Model file for the job. Use its own axes, mm. A direction names the side the tool comes from. Coordinates: 2 decimals unless noted, no trailing zeros. Order: outer loops, then holes, each group sorted by start corner. A loop starts at its lowest first (then second) coordinate and runs counter-clockwise, first axis right, second up.
from build123d import *

# Parameters (mm, degrees)
SKETCH_1_R          = 60
EXTRUDE_1_DEPTH     = 10
CHAMFER_1_SIZE      = 0.961662122
CHAMFER_1_SIZE_2    = 1
SKETCH_2_R          = 6
CUT_EXTRUDE_1_DEPTH = 10


with BuildPart() as part:
    # 草图1 → 凸台-拉伸1 (new body)
    with BuildSketch(Plane.XY):
        Circle(SKETCH_1_R)
        with BuildLine():
            Line((-38.547540209, 35.446506114), (-37.123106012, 34.236311133))
            ThreePointArc((-37.123106012, 34.236311133), (-50.5, 0), (-37.123106012, -34.236311133))
            Line((-37.123106012, -34.236311133), (-38.547540209, -35.446506114))
            ThreePointArc((-38.547540209, -35.446506114), (-38.678740931, -38.678740931), (-35.446506114, -38.547540209))
            Line((-35.446506114, -38.547540209), (-34.236311133, -37.123106012))
            ThreePointArc((-34.236311133, -37.123106012), (0, -50.5), (34.236311133, -37.123106012))
            Line((34.236311133, -37.123106012), (35.446506114, -38.547540209))
            ThreePointArc((35.446506114, -38.547540209), (38.678740931, -38.678740931), (38.547540209, -35.446506114))
            Line((38.547540209, -35.446506114), (37.123106012, -34.236311133))
            ThreePointArc((37.123106012, -34.236311133), (50.5, 0), (37.123106012, 34.236311133))
            Line((37.123106012, 34.236311133), (38.547540209, 35.446506114))
            ThreePointArc((38.547540209, 35.446506114), (38.678740931, 38.678740931), (35.446506114, 38.547540209))
            Line((35.446506114, 38.547540209), (34.236311133, 37.123106012))
            ThreePointArc((34.236311133, 37.123106012), (0, 50.5), (-34.236311133, 37.123106012))
            Line((-34.236311133, 37.123106012), (-35.446506114, 38.547540209))
            ThreePointArc((-35.446506114, 38.547540209), (-38.678740931, 38.678740931), (-38.547540209, 35.446506114))
        make_face(mode=Mode.SUBTRACT)
    extrude(amount=EXTRUDE_1_DEPTH)

    # 倒角1
    # the kernel refuses this chamfer: 1, 0.961662122 mm, written as the material it takes off along each edge
    with BuildSketch(Plane(origin=(34.236311133, 37.123106012, -2.597741643), x_dir=(-0.7418547410377812, 0.6705606185869901, 0), z_dir=(0, 0, 1)), Plane(origin=(-37.123106012, 34.236311133, -2.597741643), x_dir=(-0.6705606185869967, -0.741854741037775, 0), z_dir=(0, 0, 1)), Plane(origin=(-34.236311133, -37.123106012, -2.597741643), x_dir=(0.7418547410378011, -0.670560618586968, 0), z_dir=(0, 0, 1)), Plane(origin=(37.123106012, -34.236311133, -2.597741643), x_dir=(0.6705606185869861, 0.7418547410377846, 0), z_dir=(0, 0, 1))) as chamfer_1_piece_1:
        with BuildLine():
            Line((1.010153596, 0), (CHAMFER_1_SIZE * 0.0306993646522, -CHAMFER_1_SIZE * 0.999528663409))
            Line((CHAMFER_1_SIZE * 0.0306993646522, -CHAMFER_1_SIZE * 0.999528663409), (0, 0))
            ThreePointArc((0, 0), (0.519364344, -0.00252381), (1.010153596, 0))
        make_face()
    extrude(amount=15.195483286, mode=Mode.SUBTRACT)
    with BuildSketch(Plane(origin=(-34.236311133, 37.123106012, -2.571682988), x_dir=(-0.6474700896278034, 0.7620908627174087, 0), z_dir=(0, 0, 1)), Plane(origin=(-37.123106012, -34.236311133, -2.571682988), x_dir=(-0.7620908627174083, -0.6474700896278041, 0), z_dir=(0, 0, 1)), Plane(origin=(34.236311133, -37.123106012, -2.571682988), x_dir=(0.6474700896277805, -0.7620908627174282, 0), z_dir=(0, 0, 1)), Plane(origin=(37.123106012, 34.236311133, -2.571682988), x_dir=(0.7620908627174152, 0.6474700896277957, 0), z_dir=(0, 0, 1))) as chamfer_1_piece_2:
        with BuildLine():
            Line((CHAMFER_1_SIZE_2, 0), (0.030170276, -0.969829724))
            ThreePointArc((0.030170276, -0.969829724), (0.017838593, -0.498535983), (0, 0))
            Line((0, 0), (CHAMFER_1_SIZE_2, 0))
        make_face()
    extrude(amount=15.143365976, mode=Mode.SUBTRACT)

    # 草图2 → 切除-拉伸1 (cut)
    with BuildSketch(Plane(origin=(0, 0, 0), x_dir=(-1, 0, 0), z_dir=(0, 0, -1))):
        with Locations((60, 0)):
            Circle(SKETCH_2_R)
        with Locations((-60, 0)):
            Circle(SKETCH_2_R)
        with Locations((0, -60)):
            Circle(SKETCH_2_R)
        with Locations((0, 60)):
            Circle(SKETCH_2_R)
    extrude(amount=-CUT_EXTRUDE_1_DEPTH, mode=Mode.SUBTRACT)

    # 倒角2
    # the kernel refuses this chamfer: 2, 1.907033604 mm, written as the material it takes off along each edge
    with BuildSketch(Plane(origin=(-5.992495307, 59.7, 16.798280923), x_dir=(-0.9933125969799259, -0.11545598590369961, 0), z_dir=(0, 0, -1)), Plane(origin=(59.7, 5.992495307, 16.798280923), x_dir=(-0.11545598590369978, 0.9933125969799259, 0), z_dir=(0, 0, -1)), Plane(origin=(5.992495307, -59.7, 16.798280923), x_dir=(0.993312596979926, 0.11545598590369918, 0), z_dir=(0, 0, -1)), Plane(origin=(-59.7, -5.992495307, 16.798280923), x_dir=(0.11545598590370064, -0.9933125969799258, 0), z_dir=(0, 0, -1))) as chamfer_2_piece_1:
        with BuildLine():
            Line((1.880602566, 0), (-0.414776487, -2.618663345))
            ThreePointArc((-0.414776487, -2.618663345), (-0.066481971, -1.366902402), (0, 0))
            ThreePointArc((0, 0), (0.966657818, 0.007362718), (1.880602566, 0))
        make_face()
    extrude(amount=23.596561846, mode=Mode.SUBTRACT)
    with BuildSketch(Plane(origin=(5.992495307, 59.7, 16.798280923), x_dir=(0.9933125969799259, -0.11545598590369989, 0), z_dir=(0, 0, -1))) as chamfer_2_piece_2:
        with BuildLine():
            Line((1.880602566, 0), (-0.414776487, 2.618663345))
            ThreePointArc((-0.414776487, 2.618663345), (-0.066481971, 1.366902402), (0, 0))
            ThreePointArc((0, 0), (0.966657818, -0.007362718), (1.880602566, 0))
        make_face()
    extrude(amount=23.596561846, mode=Mode.SUBTRACT)
    with BuildSketch(Plane(origin=(-5.992495307, -59.7, 16.798280923), x_dir=(0.26943037499341854, 0.9630198715659537, 0), z_dir=(0, 0, -1)), Plane(origin=(59.7, -5.992495307, 16.798280923), x_dir=(-0.963019871565954, 0.26943037499341704, 0), z_dir=(0, 0, -1)), Plane(origin=(-59.7, 5.992495307, 16.798280923), x_dir=(0.9630198715659543, -0.26943037499341643, 0), z_dir=(0, 0, -1))) as chamfer_2_piece_3:
        with BuildLine():
            Line((2.651308592, 0), (-0.294205559, -1.857446931))
            ThreePointArc((-0.294205559, -1.857446931), (-0.158498115, -0.953603635), (0, 0))
            ThreePointArc((0, 0), (1.360472479, -0.148177801), (2.651308592, 0))
        make_face()
    extrude(amount=23.596561846, mode=Mode.SUBTRACT)


solid = part.part
Q1. Cut at A-A, the plane x = 0. List the corners of the cut face in (y, z), plus the area to 3 significant figures.
Established:
outline: (-54, 0) - (-50.5, 0) - (-50.5, 10) - (-54, 10) - close; (50.5, 0) - (54, 0) - (54, 10) - (50.5, 10) - close
area: 70.0 mm2
Q2. Which spindle directions (+Z, -Z, +X, -X, +Y, -Y) get a long thin tool onto all of the face, cutting with end or side? Do faces 1 (the face through (58.3, -6.55, 5.07)), 2 (the face through (6.587, 58.331, 5.07)), 3 (the face through (42.04, -42.81, 4.93)), 4 (the face through (0.493, 50.498, 4.93)), 5 (the face through (6.587, -58.331, 5.07)). Say none if no direction does.
Established:
face 1: +Z, -Z, +X
face 2: +Z, -Z, +Y
face 3: +Z, -Z, +X, -Y
face 4: +Z, -Z
face 5: +Z, -Z, -Y
Q3. Cut at B-B, the plane y = -28.5. List the corners of the cut face in (x, z), plus the area to 3 significant figures.
Established:
outline: (-52.8, 0) - (-41.69, 0) - (-41.69, 10) - (-52.8, 10) - close; (41.69, 0) - (52.8, 0) - (52.8, 10) - (41.69, 10) - close
area: 222 mm2
Q4. Mould opens along Y. For faces 6 (the face through (-54, 0, 5)), 7 (the face through (-58.3, 6.55, 5.07)), 8 (the face through (17, 49, 0)), 9 (the face through (-6.55, -58.3, 5.07)) say: pulls with the +Y half, pulls with the -Y half, needs draft (parallel to the pull), parting line crosses it, or undercut.
Established:
face 6: undercut
face 7: undercut
face 8: needs draft
face 9: pulls with the -Y half
Q5. Drop flat-ended pins along their axis: P1, Ø5.5, axis at x = 37.12, y = -37.12, coming from the -Z side; P2, Ø2, axis at y = -34.5, z = 3.5, coming from the -X side; P3, Ø4, axis at y = 3, z = 1, coming from the +X side; P4, Ø4, axis at y = -31, z = 2.5, coming from the +X side. Give the stop position or say it passes through.
Established:
P1: stops at z = 0
P2: stops at x = -49.78
P3: stops at x = 56.68
P4: stops at x = 52.53
Q6. Probe line 1 (X direction, y = 12.5, z = 5); line 2 (X direction, y = 27, z = 8.5); line 3 (Y direction, x = 8.5, z = 6.75). List the from-to ranges inside material, lowest first.
Established:
line 1: x = -58.68 to -48.93, 48.93 to 58.68
line 2: x = -53.58 to -42.68, 42.68 to 53.58
line 3: y = -59.39 to -49.78, 49.78 to 59.39
